```python
from build123d import *

# Parameters (mm, degrees)
CROQUIS1_R              = 60
SALIENTE_EXTRUIR1_DEPTH = 3.5
CROQUIS2_R              = 3.75
CORTAR_EXTRUIR1_DEPTH   = 3.5
MATRIZC1_COUNT          = 8
CORTAR_EXTRUIR3_REACH   = 5.5
CROQUIS4_R              = 1.92644479
CORTAR_EXTRUIR4_REACH   = 5.5
CROQUIS5_W              = 20.5
CROQUIS5_H              = 40.5


with BuildPart() as part:
    # Croquis1 → Saliente-Extruir1 (new body)
    with BuildSketch(Plane(origin=(0, 0, 0), x_dir=(1, 0, 0), z_dir=(0, 1, 0))):
        Circle(CROQUIS1_R)
    extrude(amount=SALIENTE_EXTRUIR1_DEPTH)

    # Croquis2 → Cortar-Extruir1 (cut)
    with BuildSketch(Plane(origin=(0, 3.5, 0), x_dir=(1, 0, 0), z_dir=(0, 1, 0))):
        with Locations((0, 50)):
            Circle(CROQUIS2_R)
    cortar_extruir1 = extrude(amount=-CORTAR_EXTRUIR1_DEPTH, mode=Mode.SUBTRACT)

    # MatrizC1: Cortar-Extruir1 ×8 about axis
    matrizc1_axis = Axis((0, 0, 0), (0, 1, 0))
    for i in range(1, MATRIZC1_COUNT):
        add(cortar_extruir1.rotate(matrizc1_axis, i * 360 / MATRIZC1_COUNT), mode=Mode.SUBTRACT)

    # Croquis4 → Cortar-Extruir3 (cut, up to next)
    with BuildSketch(Plane(origin=(0, 3.5, 0), x_dir=(1, 0, 0), z_dir=(0, 1, 0)), mode=Mode.PRIVATE) as cortar_extruir3_sk1:
        with Locations((5, 34)):
            Circle(CROQUIS4_R)
    cortar_extruir3_tool1 = extrude(cortar_extruir3_sk1.sketch, amount=-CORTAR_EXTRUIR3_REACH, mode=Mode.PRIVATE) & part.part
    add(cortar_extruir3_tool1.solids().sort_by_distance((5, 3.5, -34))[0], mode=Mode.SUBTRACT)
    # Croquis4 → Cortar-Extruir3 (cut, up to next)
    with BuildSketch(Plane(origin=(0, 3.5, 0), x_dir=(1, 0, 0), z_dir=(0, 1, 0)), mode=Mode.PRIVATE) as cortar_extruir3_sk2:
        with Locations((5, -16)):
            Circle(CROQUIS4_R)
    cortar_extruir3_tool2 = extrude(cortar_extruir3_sk2.sketch, amount=-CORTAR_EXTRUIR3_REACH, mode=Mode.PRIVATE) & part.part
    add(cortar_extruir3_tool2.solids().sort_by_distance((5, 3.5, 16))[0], mode=Mode.SUBTRACT)
    # Croquis4 → Cortar-Extruir3 (cut, up to next)
    with BuildSketch(Plane(origin=(0, 3.5, 0), x_dir=(1, 0, 0), z_dir=(0, 1, 0)), mode=Mode.PRIVATE) as cortar_extruir3_sk3:
        with Locations((-5, 34)):
            Circle(CROQUIS4_R)
    cortar_extruir3_tool3 = extrude(cortar_extruir3_sk3.sketch, amount=-CORTAR_EXTRUIR3_REACH, mode=Mode.PRIVATE) & part.part
    add(cortar_extruir3_tool3.solids().sort_by_distance((-5, 3.5, -34))[0], mode=Mode.SUBTRACT)
    # Croquis4 → Cortar-Extruir3 (cut, up to next)
    with BuildSketch(Plane(origin=(0, 3.5, 0), x_dir=(1, 0, 0), z_dir=(0, 1, 0)), mode=Mode.PRIVATE) as cortar_extruir3_sk4:
        with Locations((-5, -16)):
            Circle(CROQUIS4_R)
    cortar_extruir3_tool4 = extrude(cortar_extruir3_sk4.sketch, amount=-CORTAR_EXTRUIR3_REACH, mode=Mode.PRIVATE) & part.part
    add(cortar_extruir3_tool4.solids().sort_by_distance((-5, 3.5, 16))[0], mode=Mode.SUBTRACT)

    # Croquis5 → Cortar-Extruir4 (cut, up to next)
    with BuildSketch(Plane(origin=(0, 3.5, 0), x_dir=(1, 0, 0), z_dir=(0, 1, 0)), mode=Mode.PRIVATE) as cortar_extruir4_sk1:
        with Locations((0, 9)):
            Rectangle(CROQUIS5_W, CROQUIS5_H)
    cortar_extruir4_tool1 = extrude(cortar_extruir4_sk1.sketch, amount=-CORTAR_EXTRUIR4_REACH, mode=Mode.PRIVATE) & part.part
    add(cortar_extruir4_tool1.solids().sort_by_distance((0, 3.5, -9))[0], mode=Mode.SUBTRACT)


solid = part.part
```
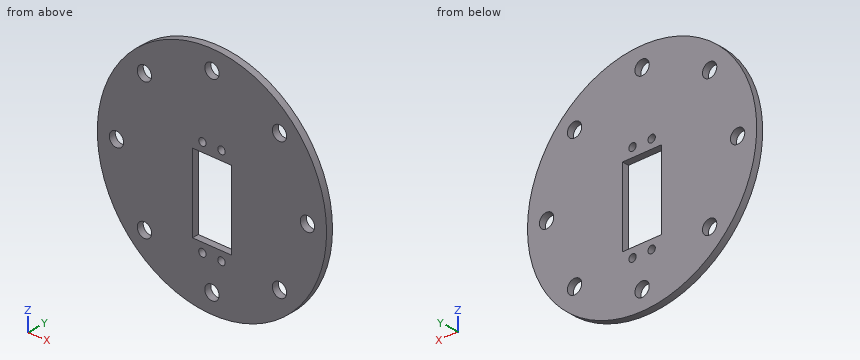
Input: part model. Units: mm. Frame: model coordinates. Coordinates: 2 decimals unless noted, no trailing zeros. Write each loop counter-clockwise with the first axis right and the second up, starting at its lowest first coordinate (ties: lowest second). Pieces come first, ordered by that corner, then holes.
1) Section A-A on z = -50. Output: boundary loops of the cut face in (x, y).
2) Section C-C on z = 36.5. Output: boundary loops of the cut face in (x, y).
3) Pin query (flat end, axial travel): pin 1 Ø1 at (y, z) = (2.5, -1.5) entering from -X; pin 2 Ø1.8 at (x, y) = (4.5, 1) entering from -Z; pin 3 Ø1 at (y, z) = (1.5, 23.5) entering from +X. Return the tip coordinate at first contact, or that it passes through.
4) Material intervals for line 1 along Z through (x, y) = (0, 1.05); line 2 along X through (y, z) = (1.65, 0); line 3 along X through (y, z) = (1.9, 33), sorted ascending.
5) Section B-B on x = 0. Output: boundary loops of the cut face in (y, z), and give its area (3 significant figures).
6) Section D-D on y = 1.45. State how many separate pieces and enclosed holes the cut face has, and give its area (3 significant figures).
Check result:
1. outline: (-33.17, 0) - (-3.75, 0) - (-3.75, 3.5) - (-33.17, 3.5) - close; (3.75, 0) - (33.17, 0) - (33.17, 3.5) - (3.75, 3.5) - close
2. outline: (-47.62, 0) - (-38.93, 0) - (-38.93, 3.5) - (-47.62, 3.5) - close; (-31.78, 0) - (31.78, 0) - (31.78, 3.5) - (-31.78, 3.5) - close; (38.93, 0) - (47.62, 0) - (47.62, 3.5) - (38.93, 3.5) - close
3. pin 1: stops at x = -59.99
3. pin 2: stops at z = -59.89
3. pin 3: stops at x = 55.42
4. line 1: z = -60 to -53.75, -46.25 to -29.25, 11.25 to 46.25, 53.75 to 60
4. line 2: x = -60 to -53.75, -46.25 to -10.25, 10.25 to 46.25, 53.75 to 60
4. line 3: x = -50.11 to -38.27, -32.44 to 32.44, 38.27 to 50.11
5. outline: (0, -60) - (3.5, -60) - (3.5, -53.75) - (0, -53.75) - close; (0, -46.25) - (3.5, -46.25) - (3.5, -29.25) - (0, -29.25) - close; (0, 11.25) - (3.5, 11.25) - (3.5, 46.25) - (0, 46.25) - close; (0, 53.75) - (3.5, 53.75) - (3.5, 60) - (0, 60) - close
5. area: 226 mm2
6. separate pieces: 1
6. enclosed holes: 13
6. area: 10,100 mm2
